Here's how the part is built. I have some questions about the finished solid (model axes, mm). A direction names the side the tool comes from. Round coordinates to 2 decimals unless told otherwise and drop trailing zeros. Write each loop counter-clockwise with the first axis right and the second up, starting at its lowest first coordinate (ties: lowest second). Pieces come first, ordered by that corner, then holes. Notation, with made-up numbers: (8, 63.5) -> (50, 63.5) arc R22 ccw to (50, 90.5) -> close; hole circle Ø4 at (68, 69.5). An arc over 180 degrees is marked (long way). Answer in a Markdown table with one row per item.
from build123d import *

# Parameters (mm, degrees)
SKETCH_R      = 25.898575
PAD_DEPTH     = 12.4
SKETCH001_R   = 19.464616
SKETCH001_R_2 = 10
PAD001_DEPTH  = 20.5
SKETCH002_R   = 16.514521
PAD002_DEPTH  = 8


with BuildPart() as part:
    # Sketch → Pad (new body)
    with BuildSketch(Plane.XY):
        Circle(SKETCH_R)
        Polygon((8.082904, 14), (-8.082904, 14), (-16.165808, 0), (-8.082904, -14), (8.082904, -14), (16.165808, 0), align=None, mode=Mode.SUBTRACT)
    extrude(amount=PAD_DEPTH)

    # Sketch001 (on Face9 of Pad) → Pad001 (join)
    with BuildSketch(Plane.XY.offset(12.4)):
        Circle(SKETCH001_R)
        Circle(SKETCH001_R_2, mode=Mode.SUBTRACT)
    extrude(amount=PAD001_DEPTH)

    # Sketch002 (on Face12 of Pad001) → Pad002 (join)
    with BuildSketch(Plane.XY.offset(32.9)):
        Circle(SKETCH002_R)
        Polygon((-6.796552, 4.737901), (-7.501419, -3.517036), (-0.704867, -8.254938), (6.796552, -4.737901), (7.501419, 3.517036), (0.704867, 8.254938), align=None, mode=Mode.SUBTRACT)
    extrude(amount=PAD002_DEPTH)


solid = part.part
1) I want a section at B-B, the plane x = 0. List the corners of the cut face in (y, z) for me.
Response:
| item | result |
|---|---|
| outline | (-25.9, 0) -> (-14, 0) -> (-14, 12.4) -> (-10, 12.4) -> (-10, 32.9) -> (-7.92, 32.9) -> (-7.92, 40.9) -> (-16.51, 40.9) -> (-16.51, 32.9) -> (-19.46, 32.9) -> (-19.46, 12.4) -> (-25.9, 12.4) -> close; (7.92, 32.9) -> (10, 32.9) -> (10, 12.4) -> (14, 12.4) -> (14, 0) -> (25.9, 0) -> (25.9, 12.4) -> (19.46, 12.4) -> (19.46, 32.9) -> (16.51, 32.9) -> (16.51, 40.9) -> (7.92, 40.9) -> close |
2) For pin 1 (3 mm diameter, centred on y = 0, z = 30, fed in from +X); pin 2 (4 mm diameter, centred on x = -0.5, z = 10.5, fed in from +Y); pin 3 (16 mm diameter, centred on x = -2, y = 4, fed in from -Z), each with a flat end and sliding along its axis, tell me the tip position at first contact or that it passes through.
Response:
| item | result |
|---|---|
| pin 1 | stops at x = 19.46 |
| pin 2 | stops at y = 25.9 |
| pin 3 | stops at z = 12.4 |
3) Which directions (+Z, -Z, +X, -X, +Y, -Y) give clear straight access to the entire face, cutting with the end or side of a thin tool? Please do faces 5 (the face through (18.566, 5.847, 22.507)), 6 (the face through (3, -7, 40.9)), 7 (the face through (7.144, -0.668, 36.844)), 8 (the face through (0, 14, 6)).
Response:
| item | result |
|---|---|
| face 5 | +Z |
| face 6 | +Z, +X, -X, +Y, -Y |
| face 7 | +Z, -Z |
| face 8 | -Z |
4) We'd pull the mould along X, two halves only. Please class faces 1 (the face through (-25.874, 1.139, 6.113)), 2 (the face through (2.993, -6.521, 36.844)), 3 (the face through (-8.7, -14.3, 32.9)), 4 (the face through (3, 10, 12.4)): +X half, -X half, draft (parallel to the pull), parting line (faces both ways), or undercut.
Response:
| item | result |
|---|---|
| face 1 | parting line |
| face 2 | undercut |
| face 3 | draft |
| face 4 | undercut |
5) I want a section at C-C, the plane y = 12. List the corners of the cut face in (x, z) for me, and give its area (3 significant figures).
Response:
| item | result |
|---|---|
| outline | (-22.95, 0) -> (-9.24, 0) -> (-9.24, 12.4) -> (9.24, 12.4) -> (9.24, 0) -> (22.95, 0) -> (22.95, 12.4) -> (15.33, 12.4) -> (15.33, 32.9) -> (11.35, 32.9) -> (11.35, 40.9) -> (-11.35, 40.9) -> (-11.35, 32.9) -> (-15.33, 32.9) -> (-15.33, 12.4) -> (-22.95, 12.4) -> close |
| area | 1,150 mm^2 |
6) I want a section at D-D, the plane z = 3. List the corners of the cut face in (x, y) for me.
Response:
| item | result |
|---|---|
| outline | circle Ø51.8 at (0, 0); hole (-16.17, 0) -> (-8.08, -14) -> (8.08, -14) -> (16.17, 0) -> (8.08, 14) -> (-8.08, 14) -> close |
7) I want a section at A-A, the plane z = 37.5. List the corners of the cut face in (x, y) for me, and give its area (3 significant figures).
Response:
| item | result |
|---|---|
| outline | circle Ø33.03 at (0, 0); hole (-7.5, -3.52) -> (-0.7, -8.25) -> (6.8, -4.74) -> (7.5, 3.52) -> (0.7, 8.25) -> (-6.8, 4.74) -> close |
| area | 678 mm^2 |
8) I need wall thicknesses on line 1 (Y direction, x = 0, z = 17.5); line 2 (Z direction, x = 5.5, y = 16); line 3 (Z direction, x = -9.5, y = 20). Which ranges of each line are inside material? Lowest first, please. Write a range as [from, to].
Response:
| item | result |
|---|---|
| line 1 | y = [-19.46, -10], [10, 19.46] |
| line 2 | z = [0, 32.9] |
| line 3 | z = [0, 12.4] |
